Design review of the part built by this model. Coordinates are the model's own, in mm. Round coordinates to 2 decimals unless told otherwise and drop trailing zeros. Write each loop counter-clockwise with the first axis right and the second up, starting at its lowest first coordinate (ties: lowest second). Pieces come first, ordered by that corner, then holes. Notation, with made-up numbers: (-35.75, 42) -> (-6.75, 42) arc R20 ccw to (-6.75, 76) -> close; hole circle Ø11 at (-13.5, 28). An arc over 180 degrees is marked (long way). One line per question, with ' | ' between items. Start each with the question number.
1) For probe 1 along Z at (x, y) = (0, -0.75); probe 2 along X at (y, z) = (-1.4, 7.5); probe 3 along Z at (x, y) = (1, 0.65), list the stretches that pass through material, from the lowest coordinate up.
2) Consider section B-B (y = 0.6). Give the boundary of the cut face in (x, z).
3) Insertion check: pin 1 Ø2.5 at (x, z) = (0, 27.5) entering from +Y; pin 2 Ø3.5 at (x, z) = (0, 7.5) entering from +Y. Each pin has a flat end and moves straight along its axis. Give the tip position at first contact, or say it passes through.
4) Consider section C-C (x = 0). Give the boundary of the cut face in (y, z).
5) Consider section D-D (z = 48). Give the boundary of the cut face in (x, y).
6) Consider section A-A (z = 7.5). Give the boundary of the cut face in (x, y).
Autodesk Inventor part; units mm, degrees
ref_plane "YZ Plane" through (0, 0, 0) normal (1, 0, 0) x (0, 1, 0)
ref_plane "XZ Plane" through (0, 0, 0) normal (0, 1, 0) x (-1, 0, 0)
ref_plane "XY Plane" through (0, 0, 0) normal (0, 0, 1) x (1, 0, 0)
sketch "スケッチ1" plane through (0, 0, 0) normal (0, 0, 1) x (1, 0, 0)
  line L0 (4.5, -2.75) -> (-4.5, -2.75)
  line L1 (-4.5, -2.75) -> (-4.5, 2.75)
  line L2 (-4.5, 2.75) -> (4.5, 2.75)
  line L3 (4.5, 2.75) -> (4.5, -2.75)
  line L4 (4.5, -2.75) -> (-4.5, 2.75) construction
  line L5 (-4.5, -2.75) -> (4.5, 2.75) construction
  point P0 (0, 0)
  dimension "d0" = 9
  dimension "d1" = 5.5
extrude "押し出し1" add sketch "スケッチ1" along normal blind 95
sketch "スケッチ2" plane through (-4.5, 2.75, 0) normal (0, 1, 0) x (1, 0, 0)
  point P0 (4.5, 0)
  point P1 (4.5, -7.5)
  point P2 (4.5, -27.5)
  point P3 (4.5, -47.5)
  point P4 (4.5, -67.5)
  point P5 (4.5, -87.5)
  dimension "d4" = 47.5
  dimension "d5" = 20
  dimension "d6" = 20
  dimension "d7" = 20
  dimension "d8" = 20
hole "穴1" at (0, 2.75, 7.5) at (0, 2.75, 27.5) at (0, 2.75, 47.5) at (0, 2.75, 67.5) at (0, 2.75, 87.5) direction (0, -1, 0) diameter 3 end through all
properties part number "slider_b5p5x9_95_sa" material "ステンレス鋼"
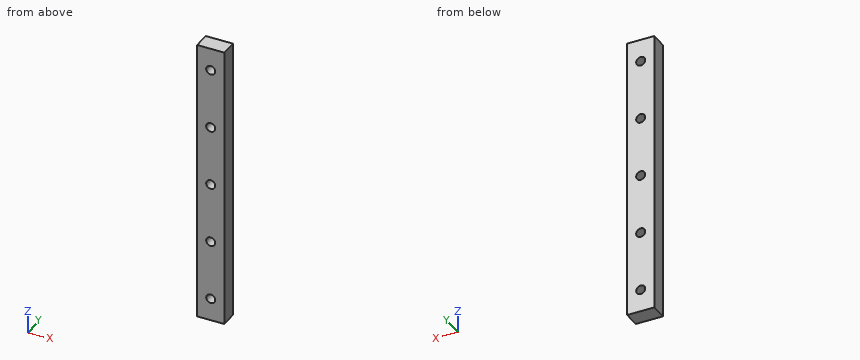
From the geometry:
1) probe 1: z = 0 to 6, 9 to 26, 29 to 46, 49 to 66, 69 to 86, 89 to 95 | probe 2: x = -4.5 to -1.5, 1.5 to 4.5 | probe 3: z = 0 to 6.38, 8.62 to 26.38, 28.62 to 46.38, 48.62 to 66.38, 68.62 to 86.38, 88.62 to 95
2) outline: (-4.5, 0) -> (4.5, 0) -> (4.5, 95) -> (-4.5, 95) -> close; hole circle Ø3 at (0, 7.5); hole circle Ø3 at (0, 27.5); hole circle Ø3 at (0, 47.5); hole circle Ø3 at (0, 67.5); hole circle Ø3 at (0, 87.5)
3) pin 1: passes through | pin 2: stops at y = 2.75
4) outline: (-2.75, 0) -> (2.75, 0) -> (2.75, 6) -> (-2.75, 6) -> close; (-2.75, 9) -> (2.75, 9) -> (2.75, 26) -> (-2.75, 26) -> close; (-2.75, 29) -> (2.75, 29) -> (2.75, 46) -> (-2.75, 46) -> close; (-2.75, 49) -> (2.75, 49) -> (2.75, 66) -> (-2.75, 66) -> close; (-2.75, 69) -> (2.75, 69) -> (2.75, 86) -> (-2.75, 86) -> close; (-2.75, 89) -> (2.75, 89) -> (2.75, 95) -> (-2.75, 95) -> close
5) outline: (-4.5, -2.75) -> (-1.41, -2.75) -> (-1.41, 2.75) -> (-4.5, 2.75) -> close; (1.41, -2.75) -> (4.5, -2.75) -> (4.5, 2.75) -> (1.41, 2.75) -> close
6) outline: (-4.5, -2.75) -> (-1.5, -2.75) -> (-1.5, 2.75) -> (-4.5, 2.75) -> close; (1.5, -2.75) -> (4.5, -2.75) -> (4.5, 2.75) -> (1.5, 2.75) -> close
